from build123d import *

# Parameters (mm, degrees)
SKETCH_1_R          = 1.6
SKETCH_1_R_2        = 3
EXTRUDE_1_DEPTH     = 3
CUT_EXTRUDE_1_REACH = 5
SKETCH_2_R          = 0.75


with BuildPart() as part:
    # 草图1 → 凸台-拉伸1 (new body)
    with BuildSketch(Plane.XY):
        with BuildLine():
            Line((2.625, 10.166581284), (19.5, 5.809475019))
            ThreePointArc((19.5, 5.809475019), (24, 0), (19.5, -5.809475019))
            Line((19.5, -5.809475019), (2.625, -10.166581284))
            ThreePointArc((2.625, -10.166581284), (-10.5, 0), (2.625, 10.166581284))
        make_face()
        with Locations((18, 0)):
            Circle(SKETCH_1_R, mode=Mode.SUBTRACT)
        Circle(SKETCH_1_R_2, mode=Mode.SUBTRACT)
    extrude(amount=EXTRUDE_1_DEPTH)

    # 草图2 → 切除-拉伸1 (cut, up to next)
    with BuildSketch(Plane.XY.offset(3), mode=Mode.PRIVATE) as cut_extrude_1_sk1:
        with Locations((0, 7.5)):
            Circle(SKETCH_2_R)
    cut_extrude_1_tool1 = extrude(cut_extrude_1_sk1.sketch, amount=-CUT_EXTRUDE_1_REACH, mode=Mode.PRIVATE) & part.part
    add(cut_extrude_1_tool1.solids().sort_by_distance((0, 7.5, 3))[0], mode=Mode.SUBTRACT)
    # 草图2 → 切除-拉伸1 (cut, up to next)
    with BuildSketch(Plane.XY.offset(3), mode=Mode.PRIVATE) as cut_extrude_1_sk2:
        with Locations((7.5, 0)):
            Circle(SKETCH_2_R)
    cut_extrude_1_tool2 = extrude(cut_extrude_1_sk2.sketch, amount=-CUT_EXTRUDE_1_REACH, mode=Mode.PRIVATE) & part.part
    add(cut_extrude_1_tool2.solids().sort_by_distance((7.5, 0, 3))[0], mode=Mode.SUBTRACT)
    # 草图2 → 切除-拉伸1 (cut, up to next)
    with BuildSketch(Plane.XY.offset(3), mode=Mode.PRIVATE) as cut_extrude_1_sk3:
        with Locations((0, -7.5)):
            Circle(SKETCH_2_R)
    cut_extrude_1_tool3 = extrude(cut_extrude_1_sk3.sketch, amount=-CUT_EXTRUDE_1_REACH, mode=Mode.PRIVATE) & part.part
    add(cut_extrude_1_tool3.solids().sort_by_distance((0, -7.5, 3))[0], mode=Mode.SUBTRACT)
    # 草图2 → 切除-拉伸1 (cut, up to next)
    with BuildSketch(Plane.XY.offset(3), mode=Mode.PRIVATE) as cut_extrude_1_sk4:
        with Locations((-7.5, 0)):
            Circle(SKETCH_2_R)
    cut_extrude_1_tool4 = extrude(cut_extrude_1_sk4.sketch, amount=-CUT_EXTRUDE_1_REACH, mode=Mode.PRIVATE) & part.part
    add(cut_extrude_1_tool4.solids().sort_by_distance((-7.5, 0, 3))[0], mode=Mode.SUBTRACT)


solid = part.part
Input: part model. Units: mm. Frame: model coordinates. Coordinates: 2 decimals unless noted, no trailing zeros. Loops run counter-clockwise (first coordinate to the right, second up) from the corner with the lowest first, then second, coordinate; pieces in that order, holes last.
(1) Section B-B on y = 0. Return the cut outline in (x, z).
(2) Section C-C on x = 18. Return the cut outline in (y, z), then the cut area to 3 significant figures.
(3) First-contact query: pin 1 Ø1.5 at (y, z) = (3, 1.5) entering from -X; pin 2 Ø1.2 at (x, y) = (0, -7.5) entering from +Z; pin 3 Ø1.5 at (x, z) = (10.5, 1.5) entering from +Y; pin 4 Ø1.5 at (y, z) = (-2, 2.5) entering from +X. Flat tips, straight axial feed; report the tip coordinate or a pass-through.
(4) Section D-D on y = -7.5. Return the cut outline in (x, z), then the cut area to 3 significant figures.
(5) Pull-direction query (Y, two-part tool) for faces 1 (the face through (-3, 0, 1)), 2 (the face through (11.181, -7.958, 1.479)), 3 (the face through (10.94, 8.02, 1.48)), 4 (the face through (-0.163, -8.232, 1.521)); classes: released by +Y, released by -Y, zero draft, split by the parting line, or undercut.
(6) Material intervals for probe 1 along X at (y, z) = (1.25, 1.65); probe 2 along Y at (x, z) = (8, 1.45); probe 3 along Y at (x, z) = (7.5, 0.5), sorted ascending.
(7) Section A-A on x = 0. Return the cut outline in (y, z).
Data:
1. outline: (-10.5, 0) - (-8.25, 0) - (-8.25, 3) - (-10.5, 3) - close; (-6.75, 0) - (-3, 0) - (-3, 3) - (-6.75, 3) - close; (3, 0) - (6.75, 0) - (6.75, 3) - (3, 3) - close; (8.25, 0) - (16.4, 0) - (16.4, 3) - (8.25, 3) - close; (19.6, 0) - (24, 0) - (24, 3) - (19.6, 3) - close
2. outline: (-6.2, 0) - (-1.6, 0) - (-1.6, 3) - (-6.2, 3) - close; (1.6, 0) - (6.2, 0) - (6.2, 3) - (1.6, 3) - close
2. area: 27.6 mm2
3. pin 1: stops at x = -10.26
3. pin 2: passes through
3. pin 3: stops at y = 8.33
3. pin 4: stops at x = 23.87
4. outline: (-7.35, 0) - (-0.75, 0) - (-0.75, 3) - (-7.35, 3) - close; (0.75, 0) - (12.95, 0) - (12.95, 3) - (0.75, 3) - close
4. area: 56.4 mm2
5. face 1: undercut
5. face 2: released by -Y
5. face 3: released by +Y
5. face 4: undercut
6. probe 1: x = -10.43 to -2.73, 2.73 to 17, 19 to 23.87
6. probe 2: y = -8.78 to -0.56, 0.56 to 8.78
6. probe 3: y = -8.91 to -0.75, 0.75 to 8.91
7. outline: (-10.5, 0) - (-8.25, 0) - (-8.25, 3) - (-10.5, 3) - close; (-6.75, 0) - (-3, 0) - (-3, 3) - (-6.75, 3) - close; (3, 0) - (6.75, 0) - (6.75, 3) - (3, 3) - close; (8.25, 0) - (10.5, 0) - (10.5, 3) - (8.25, 3) - close
